```python
from build123d import *

# Parameters (mm, degrees)
F1_DEPTH    = 22.5
F3_W        = 9.95
F3_H        = 39
F4_DEPTH    = 12.6836794258
F5_R        = 1.55
F6_DEPTH    = 4
F7_DEPTH    = 2
F8_SIZE2    = 8
F8_SIZE     = 8
F9_T1_DEPTH = 45.1469278075


# Not quite as in the source:
# - a fillet or chamfer that OpenCascade refuses, or shapes differently, is made with other operations: its cross-section is extruded or revolved along the edge and cut away or added


with BuildPart() as f1:
    # F0 (on Front) → F1 (new body, symmetric)
    with BuildSketch(Plane.XZ):
        with BuildLine():
            Line((18.5, 4), (7.0809214412, 18.555227407))
            ThreePointArc((7.0809214412, 18.555227407), (8.5067118492, 15.9386822752), (9, 13))
            ThreePointArc((9, 13), (-2.9386822752, 4.4932881508), (-7.0809214412, 18.555227407))
            Line((-7.0809214412, 18.555227407), (-18.5, 4))
            Line((-18.5, 4), (-18.5, 0))
            Line((-18.5, 0), (18.5, 0))
            Line((18.5, 0), (18.5, 4))
        make_face()
        with BuildLine():
            ThreePointArc((3, 19.9283836499), (6.3108042277, 17.1444239648), (7.55, 13))
            ThreePointArc((7.55, 13), (-4.1444239648, 6.6891957723), (-3, 19.9283836499))
            Line((-3, 19.9283836499), (-3, 21.4852813742))
            ThreePointArc((-3, 21.4852813742), (-5.2490521372, 20.3107764062), (-7.0809214412, 18.555227407))
            ThreePointArc((-7.0809214412, 18.555227407), (-2.9386822752, 4.4932881508), (9, 13))
            ThreePointArc((9, 13), (8.5067118492, 15.9386822752), (7.0809214412, 18.555227407))
            ThreePointArc((7.0809214412, 18.555227407), (5.2490521372, 20.3107764062), (3, 21.4852813742))
            Line((3, 21.4852813742), (3, 19.9283836499))
        make_face()
    extrude(amount=F1_DEPTH, both=True)

    # F3 (on offset) → F4 (cut, through all)
    with BuildSketch(Plane.XY.offset(4)):
        with Locations((-13.525, 0)):
            Rectangle(F3_W, F3_H)
        with Locations((13.525, 0)):
            Rectangle(F3_W, F3_H)
    extrude(amount=F4_DEPTH, mode=Mode.SUBTRACT)

    # F5 (on face) → F6 (cut, through all)
    with BuildSketch(Plane.XY.offset(4)):
        with Locations((14, 0)):
            Circle(F5_R)
        with Locations((-14, 0)):
            Circle(F5_R)
    extrude(amount=-F6_DEPTH, mode=Mode.SUBTRACT)

    # F5 (on face) → F7 (cut)
    with BuildSketch(Plane.XY.offset(4)):
        Polygon((11.15, 1.6454482672), (11.15, -1.6454482672), (14, -3.2908965344), (16.85, -1.6454482672), (16.85, 1.6454482672), (14, 3.2908965344), align=None)
        with Locations((14, 0)):
            Circle(F5_R, mode=Mode.SUBTRACT)
        Polygon((-11.15, -1.6454482672), (-11.15, 1.6454482672), (-14, 3.2908965344), (-16.85, 1.6454482672), (-16.85, -1.6454482672), (-14, -3.2908965344), align=None)
        with Locations((-14, 0)):
            Circle(F5_R, mode=Mode.SUBTRACT)
    extrude(amount=-F7_DEPTH, mode=Mode.SUBTRACT)

    # F8
    f8_edges = [f1.edges().sort_by_distance(p)[0] for p in [
        (-8.55, 19.5, 10.34134),
        (-8.55, -19.5, 10.34134),
        (8.55, 19.5, 10.34134),
        (8.55, -19.5, 10.34134),
    ]]
    chamfer(f8_edges, length=F8_SIZE, length2=F8_SIZE2)

    # F9: chamfer of 8 on 4 edges, made by hand

    # F9_s2 → F9_t1 (cut)
    with BuildSketch(Plane.XY.offset(-20.5734639037)):
        Polygon((-10.5, 22.5), (-18.5, 14.5), (-18.5, 22.5), align=None)
        Polygon((-10.5, -22.5), (-18.5, -14.5), (-18.5, -22.5), align=None)
        Polygon((18.5, 14.5), (10.5, 22.5), (18.5, 22.5), align=None)
        Polygon((18.5, -14.5), (10.5, -22.5), (18.5, -22.5), align=None)
    extrude(amount=F9_T1_DEPTH, mode=Mode.SUBTRACT)


solid = f1.part
```
For this review, take the finished solid that the model builds, in its own axes (mm). A direction names the side the tool comes from. Give positions to 0.01 mm unless a question says otherwise; leave off trailing zeros. Order: outer loops, then holes, each group sorted by start corner. A loop starts at its lowest first (then second) coordinate and runs counter-clockwise, first axis right, second up.
1) The part is to be moulded in two halves that separate along X. For faces 1 (the face through (-5.22, -0.32, 20.33)), 2 (the face through (-15.44, -2.46, 3.01)), 3 (the face through (18.5, 0, 2)), say which applies: released by +X, released by -X, zero draft, split by the parting line, or undercut.
2) Take a section at A-A (y = 0). State how many separate pieces and enclosed holes the cut face has, then the cut area to 3 significant figures.
3) Insertion check: pin 1 (8 mm diameter, centred on y = 15.5, z = 10.5, fed in from -X) (3 decimals); pin 2 (4 mm diameter, centred on x = -4, y = 8, fed in from -Z); pin 3 (10 mm diameter, centred on y = 3.5, z = 11, fed in from -X); pin 4 (6.5 mm diameter, centred on x = 13.5, y = 1.5, fed in from +Z). Each pin has a flat end and moves straight along its axis. Give the tip position at first contact, or say it passes through.
4) Take a section at C-C (x = 6). Give the boundary of the cut face in (y, z), then the cut area to 3 significant figures.
5) For faces 4 (the face through (-16.85, 0, 3)), 5 (the face through (11.02, 13.97, 8.84)), 6 (the face through (3, 0, 21)), list the 3-axis set-ups (+Z, -Z, +X, -X, +Y, -Y) from which the entire face can be reached by the end or side of a thin tool; tool diameter is ignored.
6) Take a section at B-B (z = 10). Give the boundary of the cut face in (x, y), then the cut area to 3 significant figures.
7) Wall thickness on line 1 (X direction, y = -4, z = 13); line 2 (X direction, y = 16.5, z = 11.75); line 3 (X direction, y = 9, z = 4.5): over which ranges is each line inside the solid? List them lowest first.
8) Take a section at D-D (y = -7). Give the boundary of the cut face in (x, z), then the cut area to 3 significant figures.
Derived:
1. face 1: released by -X
1. face 2: undercut
1. face 3: released by +X
2. separate pieces: 3
2. enclosed holes: 0
2. area: 205 mm2
3. pin 1: stops at x = -15.025
3. pin 2: stops at z = 0
3. pin 3: stops at x = -8.55
3. pin 4: stops at z = 4
4. outline: (-22.5, 0) - (22.5, 0) - (22.5, 8.42) - (-22.5, 8.42) - close; (-22.5, 17.58) - (22.5, 17.58) - (22.5, 19.71) - (-22.5, 19.71) - close
4. area: 474 mm2
5. face 4: +Z
5. face 5: +Z, +X
5. face 6: +Z, +Y, -Y
6. outline: (-13.79, -19.21) - (-10.5, -22.5) - (-6.93, -22.5) - (-6.93, 22.5) - (-10.5, 22.5) - (-13.79, 19.21) - (-13.79, 16.74) - (-8.55, 11.5) - (-8.55, -11.5) - (-13.79, -16.74) - close; (6.93, -22.5) - (10.5, -22.5) - (13.79, -19.21) - (13.79, -16.74) - (8.55, -11.5) - (8.55, 11.5) - (13.79, 16.74) - (13.79, 19.21) - (10.5, 22.5) - (6.93, 22.5) - close
6. area: 300 mm2
7. line 1: x = -8.55 to -7.55, 7.55 to 8.55
7. line 2: x = -12.42 to -7.45, 7.45 to 12.42
7. line 3: x = -8.55 to 8.55
8. outline: (-18.5, 0) - (18.5, 0) - (18.5, 4) - (8.55, 4) - (8.55, 16.68) - (7.08, 18.56) arc R9 ccw to (3, 21.49) - (3, 19.93) arc R7.55 cw (long way) to (-3, 19.93) - (-3, 21.49) arc R9 ccw to (-7.08, 18.56) - (-8.55, 16.68) - (-8.55, 4) - (-18.5, 4) - close
8. area: 240 mm2
